```python
from build123d import *

# Parameters (mm, degrees)
SKETCH6_R           = 19.175
SKETCH6_R_2         = 16
BOSS_EXTRUDE4_DEPTH = 5
BOSS_EXTRUDE5_REACH = 24.875
SKETCH7_R           = 4
BOSS_EXTRUDE6_REACH = 11.175
SKETCH8_W           = 15
SKETCH8_H           = 10


with BuildPart() as part:
    # Sketch6 → Boss-Extrude4 (new body, symmetric)
    with BuildSketch(Plane(origin=(0, 0, 0), x_dir=(1, 0, 0), z_dir=(0, 1, 0))):
        Circle(SKETCH6_R)
        Circle(SKETCH6_R_2, mode=Mode.SUBTRACT)
    extrude(amount=BOSS_EXTRUDE4_DEPTH, both=True)

    # Sketch7 → Boss-Extrude5 (add, up to next)
    with BuildSketch(Plane.XY.offset(3.7), mode=Mode.PRIVATE) as boss_extrude5_sk1:
        Circle(SKETCH7_R)
    boss_extrude5_tool1 = extrude(boss_extrude5_sk1.sketch, amount=-BOSS_EXTRUDE5_REACH, mode=Mode.PRIVATE) - part.part
    add(boss_extrude5_tool1.solids().sort_by_distance((0, 0, 3.7))[0])

    # Sketch8 → Boss-Extrude6 (add, up to next)
    with BuildSketch(Plane.XY.offset(-10), mode=Mode.PRIVATE) as boss_extrude6_sk1:
        Rectangle(SKETCH8_W, SKETCH8_H)
    boss_extrude6_tool1 = extrude(boss_extrude6_sk1.sketch, amount=-BOSS_EXTRUDE6_REACH, mode=Mode.PRIVATE) - part.part
    add(boss_extrude6_tool1.solids().sort_by_distance((0, 0, -10))[0])


solid = part.part
```
Geometry: final body of the model. Coordinates: model frame, mm. A direction names the side the tool comes from. Round coordinates to 2 decimals unless told otherwise and drop trailing zeros. Loops run counter-clockwise (first coordinate to the right, second up) from the corner with the lowest first, then second, coordinate; pieces in that order, holes last. Notation, with made-up numbers: (46, 63.5) -> (94, 63.5) arc R8 cw to (94, 77.5) -> close; hole circle Ø5 at (-6.5, 59). An arc over 180 degrees is marked (long way). Use one line per item in the form item = value.
Item 1: Draft query along Z for faces 4 (the flat face through (0, -5, -11)), 5 (the flat face through (-7.5, 0, -12)), 6 (the cylindrical face through (-4.16, 0.07, 18.72)). Return one class per face: released by +Z, released by -Z, zero draft, split by the parting line, or undercut.
Evaluation:
face_4 = zero draft
face_5 = undercut
face_6 = split by the parting line
Item 2: Access query for faces 1 (the flat face through (7.5, 0, -12)), 2 (the flat face through (0, 5, -11)), 3 (the cylindrical face through (-0.867, -3.905, -3.054)). Directions: +Z, -Z, +X, -X, +Y, -Y. A direction counts if a zero-diameter tool reaches every point of the face in a straight line with its end or side. Return the directions, or none.
Evaluation:
face_1 = +Y, -Y
face_2 = +Z, -Z, +X, -X, +Y
face_3 = none
Item 3: Material intervals for probe 1 along X at (y, z) = (0.25, 0) (3 decimals); probe 2 along Z at (x, y) = (0, 1.5) (3 decimals); probe 3 along X at (y, z) = (-0.25, -14), sorted ascending.
Evaluation:
probe_1 = -19.175 to -16, -3.992 to 3.992, 16 to 19.175
probe_2 = -19.175 to 3.7, 16 to 19.175
probe_3 = -13.1 to -7.75, -7.5 to 7.5, 7.75 to 13.1
Item 4: Cut plane D-D on z = 7.5. Output: boundary loops of the cut face in (x, y), then the cut area to 3 significant figures.
Evaluation:
outline = (-17.65, -5) -> (-14.13, -5) -> (-14.13, 5) -> (-17.65, 5) -> close; (14.13, -5) -> (17.65, -5) -> (17.65, 5) -> (14.13, 5) -> close
area = 70.3 mm2
Item 5: Cut plane B-B on x = 0. Output: boundary loops of the cut face in (y, z) (3 decimals).
Evaluation:
outline = (-5, -19.175) -> (5, -19.175) -> (5, -10) -> (4, -10) -> (4, 3.7) -> (-4, 3.7) -> (-4, -10) -> (-5, -10) -> close; (-5, 16) -> (5, 16) -> (5, 19.175) -> (-5, 19.175) -> close
Item 6: Cut plane A-A on z = 0. Output: boundary loops of the cut face in (x, y) (3 decimals).
Evaluation:
outline = (-19.175, -5) -> (-16, -5) -> (-16, 5) -> (-19.175, 5) -> close; circle Ø8 at (0, 0); (16, -5) -> (19.175, -5) -> (19.175, 5) -> (16, 5) -> close
Item 7: Cut plane C-C on y = 0. Output: boundary loops of the cut face in (x, z) (3 decimals).
Evaluation:
outline = circle Ø38.35 at (0, 0); hole (-7.5, -14.133) -> (-7.5, -10) -> (-4, -10) -> (-4, 3.7) -> (4, 3.7) -> (4, -10) -> (7.5, -10) -> (7.5, -14.133) arc R16 ccw (long way) to start
Item 8: Contact query for flat-ended pins moving along their axis: pin 1 Ø3 at (x, y) = (-1, 3) entering from -Z (3 decimals); pin 2 Ø1.2 at (y, z) = (2, -13) entering from -X; pin 3 Ø5 at (x, y) = (14, -0.5) entering from -Z. Output: stop coordinate, or through.
Evaluation:
pin_1 = -19.175
pin_2 = -14.63
pin_3 = -15.34
